Input: part model. Units: mm. Frame: model coordinates. Face numbers are marked on the shaded views. Give positions to 0.01 mm unless a question says otherwise; leave off trailing zeros. Loops run counter-clockwise (first coordinate to the right, second up) from the corner with the lowest first, then second, coordinate; pieces in that order, holes last. Notation, with made-up numbers: (-4, 36) -> (24, 36) arc R7 ccw to (24, 44) -> close; hole circle Ø1 at (-34, 59). An arc over 180 degrees is marked (long way). Answer as a JSON object with one key per item and string values. Group by question number.
```python
from build123d import *

# Parameters (mm, degrees)
SKETCH2_W           = 60
SKETCH2_H           = 50
BOSS_EXTRUDE1_DEPTH = 10
SKETCH1_R           = 3.5
CUT_EXTRUDE1_DEPTH  = 10
SKETCH3_W           = 21.5
SKETCH3_H           = 31
CUT_EXTRUDE2_DEPTH  = 1.6


with BuildPart() as part:
    # Sketch2 → Boss-Extrude1 (new body)
    with BuildSketch(Plane(origin=(0, 0, 0), x_dir=(1, 0, 0), z_dir=(0, 1, 0))):
        with Locations((30, 25)):
            Rectangle(SKETCH2_W, SKETCH2_H)
    extrude(amount=BOSS_EXTRUDE1_DEPTH)

    # Sketch1 → Cut-Extrude1 (cut)
    with BuildSketch(Plane(origin=(0, 10, 0), x_dir=(1, 0, 0), z_dir=(0, 1, 0))):
        with BuildLine():
            Line((4.6, 48.9), (4.6, 45.4))
            Line((4.6, 45.4), (1.1, 45.4))
            ThreePointArc((1.1, 45.4), (4.6, 41.9), (8.1, 45.4))
            ThreePointArc((8.1, 45.4), (7.074873734, 47.874873734), (4.6, 48.9))
        make_face()
        with BuildLine():
            Line((1.1, 45.4), (4.6, 45.4))
            Line((4.6, 45.4), (4.6, 48.9))
            ThreePointArc((4.6, 48.9), (2.125126266, 47.874873734), (1.1, 45.4))
        make_face()
        with Locations((55.4, 45.4)):
            Circle(SKETCH1_R)
        with Locations((4.6, 20)):
            Circle(SKETCH1_R)
        with Locations((55.4, 20)):
            Circle(SKETCH1_R)
    extrude(amount=-CUT_EXTRUDE1_DEPTH, mode=Mode.SUBTRACT)

    # Sketch3 → Cut-Extrude2 (cut)
    with BuildSketch(Plane(origin=(0, 10, 0), x_dir=(1, 0, 0), z_dir=(0, 1, 0))):
        with Locations((32, 21)):
            Rectangle(SKETCH3_W, SKETCH3_H)
    extrude(amount=-CUT_EXTRUDE2_DEPTH, mode=Mode.SUBTRACT)


solid = part.part
```
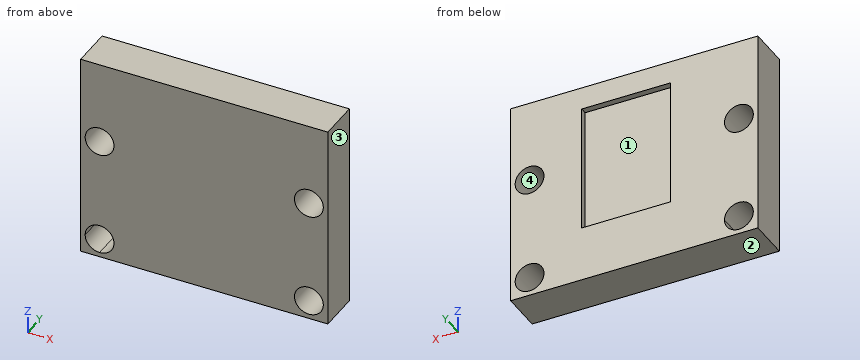
Q1. Ray query, probe 1 along Z at (x, y) = (55.4, 7.25); probe 2 along X at (y, z) = (5.75, -20); probe 3 along X at (y, z) = (6.5, -44). Return the intervals inside material, ascending.
Q2. Section A-A on x = 55.4. Return the cut outline in (y, z).
Q3. Pull-direction query (X, two-part tool) for the marked faces 1, 2, 3 and 4; classes: +X half, -X half, draft (parallel to the pull), parting line (faces both ways), or undercut.
Q4. Pin query (flat end, axial travel): pin 1 Ø9 at (x, z) = (55.4, -20) entering from -Y. Return the tip coordinate at first contact, or that it passes through.
Q5. Section D-D on z = -12.5. Return the cut outline in (x, y), then the cut area to 3 significant figures.
Q6. Section C-C on y = 5.25. Return the cut outline in (x, z), then the cut area to 3 significant figures.
Q7. Section B-B on z = -20. Return the cut outline in (x, y), then the cut area to 3 significant figures.
Numbers:
{
 "1": {"probe 1": "z = -50 to -48.9, -41.9 to -23.5, -16.5 to 0", "probe 2": "x = 0 to 1.1, 8.1 to 51.9, 58.9 to 60", "probe 3": "x = 0 to 1.39, 7.81 to 52.19, 58.61 to 60"},
 "2": {"outline": "(0, -50) -> (10, -50) -> (10, -48.9) -> (0, -48.9) -> close; (0, -41.9) -> (10, -41.9) -> (10, -23.5) -> (0, -23.5) -> close; (0, -16.5) -> (10, -16.5) -> (10, 0) -> (0, 0) -> close"},
 "3": {"face 1": "undercut", "face 2": "draft", "face 3": "+X half", "face 4": "undercut"},
 "4": {"pin 1": "stops at y = 0"},
 "5": {"outline": "(0, 0) -> (60, 0) -> (60, 10) -> (42.75, 10) -> (42.75, 8.4) -> (21.25, 8.4) -> (21.25, 10) -> (0, 10) -> close", "area": "566 mm²"},
 "6": {"outline": "(0, -50) -> (60, -50) -> (60, 0) -> (0, 0) -> close; hole circle Ø7 at (4.6, -45.4); hole circle Ø7 at (4.6, -20); hole circle Ø7 at (55.4, -45.4); hole circle Ø7 at (55.4, -20)", "area": "2,850 mm²"},
 "7": {"outline": "(0, 0) -> (1.1, 0) -> (1.1, 10) -> (0, 10) -> close; (8.1, 0) -> (51.9, 0) -> (51.9, 10) -> (42.75, 10) -> (42.75, 8.4) -> (21.25, 8.4) -> (21.25, 10) -> (8.1, 10) -> close; (58.9, 0) -> (60, 0) -> (60, 10) -> (58.9, 10) -> close", "area": "426 mm²"}
}
